```python
from build123d import *

# Parameters (mm, degrees)
SKETCH1_W           = 142.24
SKETCH1_H           = 184.15
BOSS_EXTRUDE1_DEPTH = 3.175
BOSS_EXTRUDE2_DEPTH = 50.8
SKETCH3_R           = 3.175
BOSS_EXTRUDE3_DEPTH = 152.4
SKETCH4_R           = 3.175
BOSS_EXTRUDE5_DEPTH = 47.625
SKETCH5_W           = 3.175
SKETCH5_H           = 63.808036069
BOSS_EXTRUDE6_DEPTH = 25.4


with BuildPart() as part:
    # Sketch1 → Boss-Extrude1 (new body)
    with BuildSketch(Plane(origin=(0, 0, 0), x_dir=(0, 0, -1), z_dir=(1, 0, 0))):
        with Locations((-0.521497585, -4.635193237)):
            Rectangle(SKETCH1_W, SKETCH1_H)
    extrude(amount=BOSS_EXTRUDE1_DEPTH)

    # Sketch2 → Boss-Extrude2 (add)
    with BuildSketch(Plane.ZY):
        Polygon((71.641497585, -96.710193237), (77.991497585, -96.710193237), (77.991497585, 93.789806763), (-76.948502415, 93.789806763), (-76.948502415, -96.710193237), (-70.598502415, -96.710193237), (-70.598502415, 87.439806763), (71.641497585, 87.439806763), align=None)
    extrude(amount=-BOSS_EXTRUDE2_DEPTH)

    # Sketch3 → Boss-Extrude3 (add)
    with BuildSketch(Plane(origin=(3.175, 0, 0), x_dir=(0, 0, -1), z_dir=(1, 0, 0))):
        with Locations(Location((-65.291497585, -93.535193237, 0), (0, 0, 270))):
            Circle(SKETCH3_R)
        with Locations(Location((64.248502415, -93.535193237, 0), (0, 0, 270))):
            Circle(SKETCH3_R)
    extrude(amount=BOSS_EXTRUDE3_DEPTH)

    # Sketch4 → Boss-Extrude5 (add)
    with BuildSketch(Plane(origin=(3.175, 0, 0), x_dir=(0, 0, -1), z_dir=(1, 0, 0))):
        with Locations((-36.845275585, -4.635193237)):
            Circle(SKETCH4_R)
    extrude(amount=BOSS_EXTRUDE5_DEPTH)

    # Sketch5 → Boss-Extrude6 (add)
    with BuildSketch(Plane(origin=(3.175, 0, 0), x_dir=(0, 0, -1), z_dir=(1, 0, 0))):
        with Locations((4.241002415, -10.555636975)):
            Rectangle(SKETCH5_W, SKETCH5_H)
    extrude(amount=BOSS_EXTRUDE6_DEPTH)


solid = part.part
```
The listing builds one solid part. Answer for the finished solid, in the listing's coordinates (mm). A direction names the side the tool comes from. Give positions to 0.01 mm unless a question says otherwise; leave off trailing zeros. Loops run counter-clockwise (first coordinate to the right, second up) from the corner with the lowest first, then second, coordinate; pieces in that order, holes last. Notation, with made-up numbers: (13, -22) - (39, -22) arc R18 ccw to (39, -12) - close; hole circle Ø6 at (-37, 73.5). An arc over 180 degrees is marked (long way). Return JSON: item names as keys, results as strings. Group by question number.
1. Find section D-D (y = 5). Write down the section's boundary in (x, z) (1 decimal).
2. Determine the mould class of faces 1 (the cylindrical face through (26.65, -5.85, 33.91)), 2 (the cylindrical face through (78.31, -92.85, -61.15)), 3 (the flat face through (25, 93.79, 2)), 4 (the flat face through (50.8, 91, 0)) for opening direction Y: pulls with the +Y half, pulls with the -Y half, needs draft (parallel to the pull), parting line crosses it, or undercut.
3. Given pin 1 Ø2.5 at (y, z) = (-15.5, -4.5) entering from +X (3 decimals); pin 2 Ø1 at (y, z) = (40.5, 7) entering from +X (3 decimals); pin 3 Ø1.6 at (x, z) = (12, -5) entering from -Y, each flat-ended and moving along its own axis, determine where each tip first touches the part or whether it passes through.
4. Find section C-C (z = -56.5). Write down the section's boundary in (x, y) (3 decimals), then the cut area to 3 significant figures.
5. Find section B-B (x = 24). State how many separate pieces and enclosed holes the cut face has, then the cut area to 3 significant figures.
6. Which of the six approach directions +Z, -Z, +X, -X, +Y, -Y give full straight-line access (tool end or side, diameter ignored) to faces 5 (the flat face through (16, -11, -5.829)), 6 (the flat face through (155.575, -93, -64)), 7 (the flat face through (27, 87.44, 0))?
7. Straight lines are drawn through the part: line 1 (Z direction, x = 9.5, y = -72); line 2 (Y direction, x = 37, z = 65); line 3 (Y direction, x = 39.5, z = -33.5). For each, find the intervals that lie inside material, in ascending order. Write a range as [from, to].
8. Find section A-A (y = 40). Write down the section's boundary in (x, z) (1 decimal), then the cut area to 3 significant figures.
Verdict:
{
 "1": {"outline": "(0, -76.9) - (50.8, -76.9) - (50.8, -70.6) - (3.2, -70.6) - (3.2, -5.8) - (28.6, -5.8) - (28.6, -2.7) - (3.2, -2.7) - (3.2, 71.6) - (50.8, 71.6) - (50.8, 78) - (0, 78) - close"},
 "2": {"face 1": "undercut", "face 2": "undercut", "face 3": "pulls with the +Y half", "face 4": "needs draft"},
 "3": {"pin 1": "stops at x = 28.575", "pin 2": "stops at x = 3.175", "pin 3": "stops at y = -42.46"},
 "4": {"outline": "(0, -96.71) - (3.175, -96.71) - (3.175, 87.44) - (50.8, 87.44) - (50.8, 93.79) - (0, 93.79) - close", "area": "907 mm^2"},
 "5": {"separate pieces": "5", "enclosed holes": "0", "area": "3,620 mm^2"},
 "6": {"face 5": "+X, -Y", "face 6": "+Z, -Z, +X, +Y, -Y", "face 7": "+X"},
 "7": {"line 1": "z = [-76.95, -70.6], [71.64, 77.99]", "line 2": "y = [-96.7, -90.37], [87.44, 93.79]", "line 3": "y = [87.44, 93.79]"},
 "8": {"outline": "(0, -76.9) - (50.8, -76.9) - (50.8, -70.6) - (3.2, -70.6) - (3.2, 71.6) - (50.8, 71.6) - (50.8, 78) - (0, 78) - close", "area": "1,100 mm^2"}
}
